Source: CAD feature listing. Evaluate the final solid. Frame: model axes, mm. Face numbers are marked on the shaded views. Give positions to 0.01 mm unless a question says otherwise; leave off trailing zeros. Order: outer loops, then holes, each group sorted by start corner. A loop starts at its lowest first (then second) coordinate and runs counter-clockwise, first axis right, second up. Notation, with made-up numbers: M 20.5,29.5 L 35.5,29.5 A20 ccw 35.5,47.5 Z; hole C 1,14 d1. An arc over 180 degrees is marked long. Return JSON: item names as keys, results as strings.
from build123d import *

# Parameters (mm, degrees)
F0_R     = 7
F0_R_2   = 6
F1_DEPTH = 188.96
F4_R     = 8
F5_DEPTH = 35
F9_DEPTH = 15


with BuildPart() as f1:
    # F0 (on Right) → F1 (new body)
    with BuildSketch(Plane.YZ):
        Circle(F0_R)
        Circle(F0_R_2, mode=Mode.SUBTRACT)
    extrude(amount=F1_DEPTH)

    # F4 (on face) → F5 (cut, symmetric)
    with BuildSketch(Plane(origin=(0, 0, 0), x_dir=(-0.4365976739, -0.899656863, 0), z_dir=(-0.899656863, 0.4365976739, 0))):
        Circle(F4_R)
    extrude(amount=F5_DEPTH, both=True, mode=Mode.SUBTRACT)

    # F8 (on line) → F9 (cut, symmetric)
    with BuildSketch(Plane(origin=(36.0190882591, 74.2212381898, 0), x_dir=(-0.899656863, 0.4365976739, 0), z_dir=(0.4365976739, 0.899656863, 0))):
        with BuildLine():
            ThreePointArc((-175.5327409971, 5.777498639), (-173.1401287256, -7.3576029162), (-161.999160829, 0))
            ThreePointArc((-161.999160829, 0), (-166.8581929324, 7.3576029162), (-175.5327409971, 5.777498639))
        make_face()
    extrude(amount=F9_DEPTH, both=True, mode=Mode.SUBTRACT)


solid = f1.part
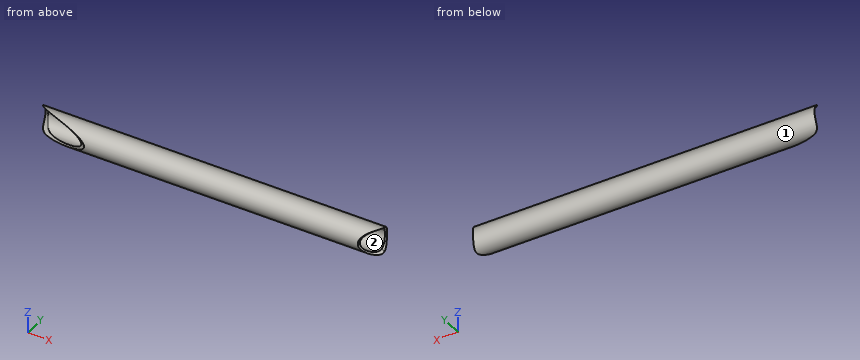
1. Draft query along Y for the marked faces 1 and 2. Return one class per face: pulls with the +Y half, pulls with the -Y half, needs draft (parallel to the pull), parting line crosses it, or undercut.
Evaluation:
{"face 1": "parting line crosses it", "face 2": "undercut"}
2. Section query B-B (x = 103). Return loops of the section in (y, z).
Evaluation:
{"outline": "C 0,0 d14; hole C 0,0 d12"}
3. First-contact query: pin 1 (6 mm diameter, centred on y = -1, z = 3.5, fed in from +X); pin 2 (4 mm diameter, centred on x = 75, y = -4.5, fed in from +Z); pin 3 (4 mm diameter, centred on x = 160, y = 3, fed in from -Z). Flat tips, straight axial feed; report the tip coordinate or a pass-through.
Evaluation:
{"pin 1": "stops at x = 183.52", "pin 2": "stops at z = 6.54", "pin 3": "stops at z = -6.93"}
4. Section query A-A (z = -2.25). Return loops of the section in (x, y).
Evaluation:
{"outline": "M 3.93,6.63 L 6.12,5.56 L 183.13,5.56 L 183.64,6.63 Z; M 29.05,-5.56 L 31.24,-6.63 L 177.21,-6.63 L 177.73,-5.56 Z"}
5. Ray query, probe 1 along Z at (x, y) = (56, 0); probe 2 along Y at (x, z) = (83.5, 1.75). Return the intervals inside material, ascending.
Evaluation:
{"probe 1": "z = -7 to -6, 6 to 7", "probe 2": "y = -6.78 to -5.74, 5.74 to 6.78"}
